Autodesk Inventor part; units mm, degrees
ref_plane "YZ Plane" through (0, 0, 0) normal (1, 0, 0) x (0, 1, 0)
ref_plane "XZ Plane" through (0, 0, 0) normal (0, 1, 0) x (-1, 0, 0)
ref_plane "XY Plane" through (0, 0, 0) normal (0, 0, 1) x (1, 0, 0)
sketch "Sketch1" plane through (0, 0, 0) normal (0, 1, 0) x (-1, 0, 0)
  circle A0 centre (0, 0) radius 62.5
  circle A1 centre (0, 0) radius 53
  circle A2 centre (0, -53) radius 4.05
  circle A3 centre (0, 0) radius 44
  circle A4 centre (45.8993, -26.5) radius 4.05
  circle A5 centre (45.8993, 26.5) radius 4.05
  circle A6 centre (0, 53) radius 4.05
  circle A7 centre (-45.8993, 26.5) radius 4.05
  circle A8 centre (-45.8993, -26.5) radius 4.05
  dimension "d1" = 106
  dimension "d0" = 125
  dimension "d4" = 360
  dimension "d18" = 8.1
extrude "Extrusion1" add sketch "Sketch1" along normal blind 12 contours A0 | A1 A4 A2 A8 A7 A6 A5
sketch "Sketch2" plane through (0, 12, 0) normal (0, 1, 0) x (1, 0, 0)
  circle A0 centre (0, 0) radius 44
  circle A1 centre (0, 0) radius 15
  circle A2 centre (-22, 0) radius 4.05
  circle A3 centre (-11, -19.0526) radius 4.05
  circle A4 centre (11, -19.0526) radius 4.05
  circle A5 centre (22, 0) radius 4.05
  circle A6 centre (11, 19.0526) radius 4.05
  circle A7 centre (-11, 19.0526) radius 4.05
  dimension "d8" = 30
  dimension "d11" = 22
  dimension "d12" = 8.1
  dimension "d15" = 360
extrude "Extrusion2" add sketch "Sketch2" against normal blind 8
sketch "Sketch3" plane through (0, 12, 0) normal (0, 1, 0) x (1, 0, 0)
  circle A0 centre (0, 0) radius 30
  circle A1 centre (0, 0) radius 15
  circle A2 centre (-22, 0) radius 4.05
  circle A3 centre (-11, -19.0526) radius 4.05
  circle A4 centre (11, -19.0526) radius 4.05
  circle A5 centre (22, 0) radius 4.05
  circle A6 centre (11, 19.0526) radius 4.05
  circle A7 centre (-11, 19.0526) radius 4.05
  circle A8 centre (0, 0) radius 62.5
  circle A9 centre (0, 53) radius 4.05
  circle A10 centre (-45.8993, 26.5) radius 4.05
  circle A11 centre (-45.8993, -26.5) radius 4.05
  circle A12 centre (0, -53) radius 4.05
  circle A13 centre (45.8993, -26.5) radius 4.05
  circle A14 centre (45.8993, 26.5) radius 4.05
  dimension "d17" = 60
extrude "Extrusion3" add sketch "Sketch3" along normal blind 24 contours A0
sketch "Sketch4" plane through (0, 12, 0) normal (0, 1, 0) x (1, 0, 0)
  circle A0 centre (0, 0) radius 46.75
  circle A1 centre (0, 0) radius 44
  circle A2 centre (0, 0) radius 30
  circle A3 centre (0, 0) radius 62.5
  circle A4 centre (0, 53) radius 4.05
  circle A5 centre (-45.8993, 26.5) radius 4.05
  circle A6 centre (-45.8993, -26.5) radius 4.05
  circle A7 centre (0, -53) radius 4.05
  circle A8 centre (45.8993, -26.5) radius 4.05
  circle A9 centre (45.8993, 26.5) radius 4.05
  dimension "d24" = 93.5
extrude "Extrusion4" add sketch "Sketch4" along normal blind 11 contours A0 | A1
sketch "Sketch5" plane through (0, 36, 0) normal (0, 1, 0) x (1, 0, 0)
  circle A0 centre (0, 0) radius 30
  circle A1 centre (-11, 19.0526) radius 4.05
  circle A2 centre (11, 19.0526) radius 4.05
  circle A3 centre (22, 0) radius 4.05
  circle A4 centre (11, -19.0526) radius 4.05
  circle A5 centre (-11, -19.0526) radius 4.05
  circle A6 centre (-22, 0) radius 4.05
  circle A7 centre (0, 0) radius 15
extrude "Extrusion5" add sketch "Sketch5" along normal blind 2
properties part number "OnPatronFlanech"
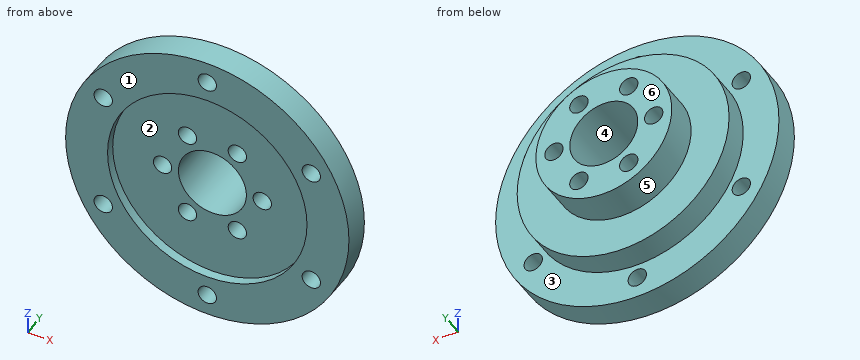
Model file for the job. Use its own axes, mm. Face numbers are marked on the shaded views. A direction names the side the tool comes from. Coordinates: 2 decimals unless noted, no trailing zeros. Write each loop counter-clockwise with the first axis right and the second up, starting at its lowest first coordinate (ties: lowest second). Pieces come first, ordered by that corner, then holes. Notation, with made-up numbers: (31, 60.25) - (89, 60.25) arc R10 cw to (89, 70.25) - close; hole circle Ø4 at (52, 26). An arc over 180 degrees is marked (long way). Use a Markdown table: item, result. Add a question column.
Item 1: Two-plate mould, pull along Z, no slides. Class the marked faces 4, 5 and 6: pulls with the +Z half, pulls with the -Z half, needs draft (parallel to the pull), parting line crosses it, or undercut.
Item 2: Drill centre lines: line 1 along X through (y, z) = (26, 0); line 2 along Z through (x, y) = (-10, 5.5); line 3 along X through (y, z) = (10, 19). Where is each one in solid material? Low to high.
Item 3: Band-saw the part on A-A, the plane x = 0. Write the cut outline in (y, z), and give its area (3 significant figures).
Item 4: Band-saw the part on B-B, the plane y = 33.5. Write the cut outline in (x, z).
Item 5: Band-saw the part on D-D, the plane z = 53. Write the cut outline in (x, y), and give its area (3 significant figures).
Item 6: Band-saw the part on C-C, the plane z = -26.5. Write the cut outline in (x, y), and give its area (3 significant figures).
Item 7: 3-axis set-ups, long thin cutter, end or side, ignore diameter. For the marked faces 1, 2 and 3: which of +Z, -Z, +X, -X, +Y, -Y reach the whole face in a straight line?
Item 8: Drop flat-ended pins along their axis: pin 1 (10.5 mm diameter, centred on x = -45.9, z = -26.5, fed in from +Y); pin 2 (8 mm diameter, centred on x = 31, y = 13.5, fed in from -Z); pin 3 (10 mm diameter, centred on y = 19, z = 32, fed in from +X); pin 4 (4 mm diameter, centred on x = 41, z = 41, fed in from -Y). Give the stop position or say it passes through.
A:
| question | item | result |
|---|---|---|
| 1 | face 4 | undercut |
| 1 | face 5 | parting line crosses it |
| 1 | face 6 | needs draft |
| 2 | line 1 | x = -30 to -26.05, -17.95 to -15, 15 to 17.95, 26.05 to 30 |
| 2 | line 2 | z = -61.69 to -22.98, -15.13 to -11.18, 11.18 to 15.13, 22.98 to 61.69 |
| 2 | line 3 | x = -59.54 to -15.05, -6.95 to 6.95, 15.05 to 59.54 |
| 3 | outline | (0, -62.5) - (12, -62.5) - (12, -57.05) - (0, -57.05) - close; (0, -48.95) - (12, -48.95) - (12, -46.75) - (23, -46.75) - (23, -30) - (38, -30) - (38, -15) - (4, -15) - (4, -44) - (0, -44) - close; (0, 44) - (4, 44) - (4, 15) - (38, 15) - (38, 30) - (23, 30) - (23, 46.75) - (12, 46.75) - (12, 48.95) - (0, 48.95) - close; (0, 57.05) - (12, 57.05) - (12, 62.5) - (0, 62.5) - close |
| 3 | area | 1,860 mm² |
| 4 | outline | circle Ø60 at (0, 0); hole circle Ø8.1 at (-22, 0); hole circle Ø8.1 at (-11, -19.05); hole circle Ø8.1 at (-11, 19.05); hole circle Ø30 at (0, 0); hole circle Ø8.1 at (11, -19.05); hole circle Ø8.1 at (11, 19.05); hole circle Ø8.1 at (22, 0) |
| 5 | outline | (-33.12, 0) - (-4.05, 0) - (-4.05, 12) - (-33.12, 12) - close; (4.05, 0) - (33.12, 0) - (33.12, 12) - (4.05, 12) - close |
| 5 | area | 698 mm² |
| 6 | outline | (-56.6, 0) - (-49.95, 0) - (-49.95, 12) - (-56.6, 12) - close; (-41.85, 0) - (-35.12, 0) - (-35.12, 4) - (35.12, 4) - (35.12, 0) - (41.85, 0) - (41.85, 12) - (38.51, 12) - (38.51, 23) - (14.06, 23) - (14.06, 38) - (-14.06, 38) - (-14.06, 23) - (-38.51, 23) - (-38.51, 12) - (-41.85, 12) - close; (49.95, 0) - (56.6, 0) - (56.6, 12) - (49.95, 12) - close |
| 6 | area | 2,150 mm² |
| 7 | face 1 | +Z, -Z, +X, -X, -Y |
| 7 | face 2 | -Y |
| 7 | face 3 | +Y |
| 8 | pin 1 | stops at y = 12 |
| 8 | pin 2 | stops at z = -56.23 |
| 8 | pin 3 | stops at x = 38.16 |
| 8 | pin 4 | stops at y = 0 |
